Can you work these out from the model? Positions are in its coordinate system, mm. Give positions to 0.01 mm unless a question says otherwise; leave off trailing zeros. Order: outer loops, then holes, each group sorted by start corner. A loop starts at its lowest first (then second) coordinate and runs counter-clockwise, first axis right, second up.
Item 1: I want a section at A-A, the plane z = -33.88. Write out the boundary of the cut face in (x, y) (3 decimals), then the cut area to 3 significant figures.
Item 2: If I drill on line 1 along X through (y, z) = (2.5, 28.5) (3 decimals); line 2 along Z through (x, y) = (4.5, 2); line 3 along Y through (x, z) = (-30.35, 33.88), over which ranges is the centre line in solid material (lowest first)?
Item 3: I want a section at B-B, the plane x = 14. Write out the boundary of the cut face in (y, z), then the cut area to 3 significant figures.
Item 4: I want a section at C-C, the plane z = 29. Write out the boundary of the cut face in (x, y) (3 decimals), then the cut area to 3 significant figures.
Item 5: I want a section at D-D, the plane y = 4. Count the separate pieces of the cut face and the enclosed holes in it, then the cut area to 3 significant figures.
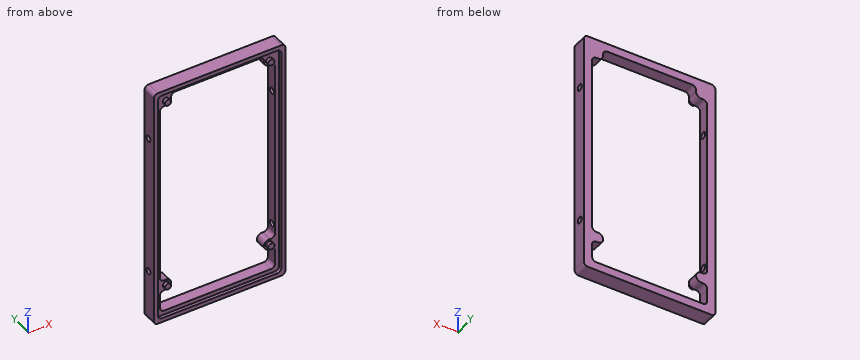
Autodesk Inventor part; units mm, degrees
ref_plane "YZ Plane" through (0, 0, 0) normal (1, 0, 0) x (0, 1, 0)
ref_plane "XZ Plane" through (0, 0, 0) normal (0, 1, 0) x (-1, 0, 0)
ref_plane "XY Plane" through (0, 0, 0) normal (0, 0, 1) x (1, 0, 0)
sketch "Sketch1" plane through (0, 0, 0) normal (0, 1, 0) x (-1, 0, 0)
  line L0 (29.575, 58.88) -> (-29.575, 58.88)
  line L1 (-31.575, 56.88) -> (-31.575, -56.88)
  line L2 (-29.575, -58.88) -> (29.575, -58.88)
  line L3 (31.575, -56.88) -> (31.575, 56.88)
  line L4 (21.765, 52.07) -> (27.765, 52.07) construction
  line L5 (0, 0) -> (-80.4548, 0) construction
  line L6 (0, 0) -> (0, 46.6746) construction
  line L7 (28.575, 55.88) -> (-28.575, 55.88) construction
  line L8 (-28.575, 55.88) -> (-28.575, -55.88) construction
  line L9 (-28.575, -55.88) -> (28.575, -55.88) construction
  line L10 (28.575, -55.88) -> (28.575, 55.88) construction
  circle A0 centre (24.765, 52.07) radius 1.5 construction
  circle A1 centre (-24.765, 52.07) radius 1.5 construction
  circle A2 centre (24.765, -41.91) radius 3.8303 construction
  circle A3 centre (-24.765, -41.91) radius 3.8303 construction
  line L11 (20.265, 54.88) -> (-20.265, 54.88)
  line L12 (-25.575, -54.88) -> (25.575, -54.88)
  line L13 (28.575, 55.88) -> (-28.575, -55.88) construction
  line L14 (28.575, -55.88) -> (-28.575, 55.88) construction
  arc A4 (25.575, -54.88) -> (27.575, -52.88) centre (25.575, -52.88) ccw
  arc A5 (-27.575, -52.88) -> (-25.575, -54.88) centre (-25.575, -52.88) ccw
  arc A6 (-29.575, 58.88) -> (-31.575, 56.88) centre (-29.575, 56.88) ccw
  arc A7 (31.575, 56.88) -> (29.575, 58.88) centre (29.575, 56.88) ccw
  arc A8 (29.575, -58.88) -> (31.575, -56.88) centre (29.575, -56.88) ccw
  arc A9 (-31.575, -56.88) -> (-29.575, -58.88) centre (-29.575, -56.88) ccw
  circle A10 centre (24.765, 52.07) radius 1.5
  line L15 (24.765, 49.57) -> (25.575, 49.57)
  line L16 (22.265, 52.07) -> (22.265, 52.88)
  arc A11 (27.575, 47.57) -> (25.575, 49.57) centre (25.575, 47.57) ccw
  arc A12 (22.265, 52.88) -> (20.265, 54.88) centre (20.265, 52.88) ccw
  circle A13 centre (-24.765, 52.07) radius 1.5 construction
  circle A14 centre (-24.765, 52.07) radius 1.5
  arc A15 (-24.765, 49.57) -> (-22.265, 52.07) centre (-24.765, 52.07) ccw
  arc A16 (-25.575, 49.57) -> (-27.575, 47.57) centre (-25.575, 47.57) ccw
  arc A17 (-20.265, 54.88) -> (-22.265, 52.88) centre (-20.265, 52.88) ccw
  line L17 (-24.765, 49.57) -> (-25.575, 49.57)
  line L18 (-22.265, 52.07) -> (-22.265, 52.88)
  arc A18 (22.265, 52.07) -> (24.765, 49.57) centre (24.765, 52.07) ccw
  circle A19 centre (24.765, -41.91) radius 1.5
  circle A20 centre (-24.765, -41.91) radius 1.5
  arc A21 (-24.765, -44.41) -> (-24.765, -39.41) centre (-24.765, -41.91) ccw
  line L19 (-24.765, -44.41) -> (-25.575, -44.41)
  line L20 (-24.765, -39.41) -> (-25.575, -39.41)
  line L21 (-27.575, 47.57) -> (-27.575, -37.41)
  line L22 (-27.575, -46.41) -> (-27.575, -52.88)
  arc A22 (-27.575, -37.41) -> (-25.575, -39.41) centre (-25.575, -37.41) ccw
  arc A23 (-25.575, -44.41) -> (-27.575, -46.41) centre (-25.575, -46.41) ccw
  line L23 (24.765, -44.41) -> (25.575, -44.41)
  line L24 (24.765, -39.41) -> (25.575, -39.41)
  arc A24 (25.575, -39.41) -> (27.575, -37.41) centre (25.575, -37.41) ccw
  arc A25 (27.575, -46.41) -> (25.575, -44.41) centre (25.575, -46.41) ccw
  line L25 (27.575, -52.88) -> (27.575, -46.41)
  line L26 (27.575, -37.41) -> (27.575, 47.57)
  arc A26 (24.765, -39.41) -> (24.765, -44.41) centre (24.765, -41.91) ccw
  point P0 (31.575, 58.88)
  point P1 (-31.575, -58.88)
  point P2 (-31.575, 58.88)
  point P3 (31.575, -58.88)
  point P4 (-27.575, 54.88)
  dimension "d77" = 57.15
  dimension "d78" = 3.81
  dimension "d79" = 3.81
  dimension "d80" = 3.81
  dimension "d81" = 3.81
  dimension "d82" = 3
  dimension "d85" = 111.76
  dimension "d88" = 3.81
  dimension "d100" = 1
  dimension "d101" = 3
  dimension "d104" = 1
  dimension "d107" = 3
  dimension "d109" = 3
  dimension "d122" = 3
  dimension "d123" = 2
  dimension "d132" = 2
  dimension "d145" = 2
  dimension "d150" = 2.5
  dimension "d151" = 3
  dimension "d152" = 3
  dimension "d154" = 5
  dimension "d155" = 2
  dimension "d156" = 1
  dimension "d157" = 12.97
extrude "Extrusion1" add sketch "Sketch1" along normal blind 7
sketch "Sketch2" plane through (0, 0, 0) normal (0, -1, 0) x (1, 0, 0)
  line L0 (-27.575, 56.88) -> (27.575, 56.88)
  line L1 (29.575, 54.88) -> (29.575, -54.88)
  line L2 (27.575, -56.88) -> (-27.575, -56.88)
  line L3 (-29.575, -54.88) -> (-29.575, 54.88)
  line L4 (29.575, 56.88) -> (-29.575, -56.88) construction
  line L5 (29.575, -56.88) -> (-29.575, 56.88) construction
  arc A0 (29.575, 54.88) -> (27.575, 56.88) centre (27.575, 54.88) ccw
  arc A1 (-27.575, 56.88) -> (-29.575, 54.88) centre (-27.575, 54.88) ccw
  arc A2 (-29.575, -54.88) -> (-27.575, -56.88) centre (-27.575, -54.88) ccw
  arc A3 (27.575, -56.88) -> (29.575, -54.88) centre (27.575, -54.88) ccw
  circle A4 centre (-24.765, 52.07) radius 1.5
  point P0 (0, 0)
  dimension "d26" = 59.15
  dimension "d27" = 113.76
  dimension "d131" = 2
extrude "Extrusion2" cut sketch "Sketch2" against normal blind 1.6
sketch "Sketch5" plane through (-31.575, 0, -56.88) normal (-1, 0, 0) x (0, 0, 1)
  circle A0 centre (23, 4) radius 1.5
  circle A1 centre (90.76, 4) radius 1.5
  line L0 (10.47, 7) -> (4, 7)
  line L1 (115.76, 0) -> (115.76, 7)
  line L2 (-2, 0) -> (-2, 7)
  circle A2 centre (90.76, 5.5) radius 1.5
  line L3 (92.26, 4) -> (92.26, 5.5)
  line L4 (90.76, 4) -> (90.76, 5.5) construction
  line L5 (89.26, 5.5) -> (89.26, 4)
  point P0 (56.88, 0)
  point P1 (109.76, 7)
  point P2 (104.45, 7)
  dimension "d133" = 3
  dimension "d134" = 3
  dimension "d135" = 3
  dimension "d136" = 3
  dimension "d137" = 25
  dimension "d138" = 25
  dimension "d141" = 3
  dimension "d142" = 1.5
extrude "Extrusion5" cut sketch "Sketch5" against normal blind 70 contours A0 | A1 A2 | A1 A2 picked at (90.702, 3.0107) picked at (90.702, 4.5034)
sketch "Sketch6" plane through (0, 1.6, 0) normal (0, -1, 0) x (1, 0, 0)
  circle A0 centre (-24.765, 52.07) radius 1.5
  circle A1 centre (24.765, 52.07) radius 1.5
  circle A2 centre (24.765, -41.91) radius 1.5
  circle A3 centre (-24.765, -41.91) radius 1.5
  point P0 (0, 0)
extrude "Extrusion6" add sketch "Sketch6" along normal blind 1.6 and the other way blind 5.4
properties part number "RahmenV05_BOT"
Results list:
1. outline: (-31.575, 0) - (-29.575, 0) - (-29.575, 1.6) - (-27.575, 1.6) - (-27.575, 2.5) - (-31.575, 2.5) - close; (-31.575, 5.5) - (-27.575, 5.5) - (-27.575, 7) - (-31.575, 7) - close; (27.575, 1.6) - (29.575, 1.6) - (29.575, 0) - (31.575, 0) - (31.575, 2.5) - (27.575, 2.5) - close; (27.575, 5.5) - (31.575, 5.5) - (31.575, 7) - (27.575, 7) - close
1. area: 25.6 mm2
2. line 1: x = -31.575 to -27.575, 27.575 to 31.575
2. line 2: z = -58.88 to -54.88, 54.88 to 58.88
2. line 3: y = 0 to 2.5, 5.5 to 7
3. outline: (0, -58.88) - (7, -58.88) - (7, -54.88) - (1.6, -54.88) - (1.6, -56.88) - (0, -56.88) - close; (0, 56.88) - (1.6, 56.88) - (1.6, 54.88) - (7, 54.88) - (7, 58.88) - (0, 58.88) - close
3. area: 49.6 mm2
4. outline: (-31.575, 0) - (-29.575, 0) - (-29.575, 1.6) - (-27.575, 1.6) - (-27.575, 7) - (-31.575, 7) - close; (27.575, 1.6) - (29.575, 1.6) - (29.575, 0) - (31.575, 0) - (31.575, 7) - (27.575, 7) - close
4. area: 49.6 mm2
5. separate pieces: 4
5. enclosed holes: 0
5. area: 1,440 mm2
